Here's how the part is built. I have some questions about the finished solid (model axes, mm). A direction names the side the tool comes from. Coordinates: 2 decimals unless noted, no trailing zeros. Write each loop counter-clockwise with the first axis right and the second up, starting at its lowest first coordinate (ties: lowest second). Pieces come first, ordered by that corner, then holes. Notation, with made-up numbers: (22, -15) -> (41, -15) arc R25 cw to (41, 16) -> close; hole circle Ø7 at (8.5, 74.25). An arc over 180 degrees is marked (long way). Put each result on its own line as item: value.
```python
from build123d import *

# Parameters (mm, degrees)
EXTRUDE_1_DEPTH     = 1
SKETCH_3_R          = 2
EXTRUDE_2_DEPTH     = 2
SKETCH_4_W          = 36.891891892
SKETCH_4_H          = 44.115479116
SKETCH_4_W_2        = 11
SKETCH_4_H_2        = 11
CUT_EXTRUDE_1_DEPTH = 14


with BuildPart() as part:
    # Sketch 1 → Revolve 1 (revolve)
    with BuildSketch(Plane(origin=(0, 0, 0), x_dir=(0, 0, -1), z_dir=(1, 0, 0)), mode=Mode.PRIVATE) as revolve_1_sk:
        Polygon((-34.571428571, 0), (-34.571428571, 18.260869565), (-38, 18.260869565), (-38, 21), (-34, 21), (-34, 20), (-14, 20), (-14, 7.586206897), (-8.4, 7.586206897), (-8.4, 5.001506871), (-0.600035703, 4.757745806), (0, 4.157710103), (0, 0), align=None)
    revolve(revolve_1_sk.sketch.rotate(Axis((0, 0, 0), (0, 0, 1)), 270), axis=Axis((0, 0, 0), (0, 0, 1)))

    # Sketch 2 → Extrude 1 (add)
    with BuildSketch(Plane.XY.offset(34.571428571)):
        Polygon((-11.879393924, -11.879393924), (6.135636089, 4.341411958), (5.656854249, 5.656854249), (4.341411958, 6.135636089), align=None)
    extrude(amount=EXTRUDE_1_DEPTH)

    # Sketch 3 → Extrude 2 (add)
    with BuildSketch(Plane.XY.offset(34.571428571)):
        with Locations(Location((0, 0, 0), (0, 0, 201.92023219))):
            Circle(SKETCH_3_R)
    extrude(amount=EXTRUDE_2_DEPTH)

    # Sketch 4 → Cut-Extrude 1 (cut)
    with BuildSketch(Plane.XY):
        with Locations((-1.160933661, -1.547911548)):
            Rectangle(SKETCH_4_W, SKETCH_4_H)
        Rectangle(SKETCH_4_W_2, SKETCH_4_H_2, mode=Mode.SUBTRACT)
    extrude(amount=CUT_EXTRUDE_1_DEPTH, mode=Mode.SUBTRACT)


solid = part.part
```
Item 1: Imagine slicing it at B-B on y = -16. Write out the boundary of the cut face in (x, z), then the cut area to 3 significant figures.
Output:
outline: (-13.6, 34) -> (-12, 34) -> (-12, 14) -> (12, 14) -> (12, 34) -> (13.6, 34) -> (13.6, 38) -> (8.8, 38) -> (8.8, 34.57) -> (-8.8, 34.57) -> (-8.8, 38) -> (-13.6, 38) -> close
area: 528 mm²
Item 2: Imagine slicing it at C-C on x = -17.5. Write out the boundary of the cut face in (y, z).
Output:
outline: (-11.61, 34) -> (-9.68, 34) -> (-9.68, 14) -> (9.68, 14) -> (9.68, 34) -> (11.61, 34) -> (11.61, 38) -> (5.22, 38) -> (5.22, 34.57) -> (-5.22, 34.57) -> (-5.22, 38) -> (-11.61, 38) -> close
Item 3: Which directions (+Z, -Z, +X, -X, +Y, -Y) give clear straight access to the entire face, cutting with the end or side of a thin tool? Please do faces 5 (the flat face through (0, -5.5, 11)), 6 (the flat face through (9, 0, 14)), 7 (the flat face through (-6.391, -6.938, 35.064)).
Output:
face 5: -Z, +X, -X, -Y
face 6: -Z
face 7: +Z
Item 4: For P1, Ø4.5, axis at y = 1, z = 12, coming from the -X side; P2, Ø3, axis at x = 2, y = 2, coming from the +Z side; P3, Ø2, axis at y = 4, z = 9.5, coming from the +X side; P4, Ø6, axis at y = 9, z = 5, coming from the +X side, each with a flat end and sliding along its axis, tell me the tip position at first contact or that it passes through.
Output:
P1: stops at x = -20
P2: stops at z = 36.57
P3: stops at x = 5.5
P4: passes through
Item 5: Please list where these lines run through material, in increasing order: line 1 along Y through (x, z) = (0, 36.4); line 2 along Y through (x, z) = (0, 37.1); line 3 along Z through (x, y) = (8, 16.5). Write a range as from..to.
Output:
line 1: y = -21..-18.26, -2..2, 18.26..21
line 2: y = -21..-18.26, 18.26..21
line 3: z = 14..38
Item 6: Imagine slicing it at A-A on z = 11.5. Write out the boundary of the cut face in (x, y) (3 decimals), then the cut area to 3 significant figures.
Output:
outline: (-5.5, -5.225) arc R7.586 ccw to (-5.225, -5.5) -> (5.225, -5.5) arc R7.586 ccw to (5.5, -5.225) -> (5.5, 5.225) arc R7.586 ccw to (5.225, 5.5) -> (-5.225, 5.5) arc R7.586 ccw to (-5.5, 5.225) -> close
area: 121 mm²
Item 7: If we mould it in two halves opening along X, with no side actions, what happens to faces 1 (the flat face through (5.5, 0, 11)), 2 (the flat face through (19, -8, 34)), 3 (the flat face through (2.47, 4.06, 35.06)), 4 (the flat face through (-5, -5, 35.571))? For each: released by +X, released by -X, zero draft, split by the parting line, or undercut.
Output:
face 1: released by +X
face 2: zero draft
face 3: undercut
face 4: undercut
Item 8: Imagine slicing it at D-D on z = 23.5. Write out the boundary of the cut face in (x, y).
Output:
outline: circle Ø40 at (0, 0)
